from build123d import *

# Parameters (mm, degrees)
IZIM1_W                     = 20
IZIM1_H                     = 20
Y_KSEKLIK_EKSTR_ZYON1_DEPTH = 10
BO_ALTMA1_T                 = -1
IZIM2_R                     = 20
KES_EKSTR_ZYON1_DEPTH       = 29
Y_KSEKLIK_EKSTR_ZYON2_DEPTH = 4
Y_KSEKLIK_EKSTR_ZYON3_REACH = 29.441
IZIM4_W                     = 8
IZIM4_H                     = 1.735346843
Y_KSEKLIK_EKSTR_ZYON4_START = -10.860571
IZIM6_W                     = 1.735346843
IZIM6_H                     = 8
Y_KSEKLIK_EKSTR_ZYON4_DEPTH = 10.860571
BO_ALTMA2_START             = 1.404082058
BO_ALTMA2_OUTLINE_W         = 9.860571099
BO_ALTMA2_OUTLINE_H         = 6
BO_ALTMA2_DEPTH             = 9.595917942
BO_ALTMA2_START_2           = 10
BO_ALTMA2_2_OUTLINE_W       = 1.735346843
BO_ALTMA2_2_OUTLINE_H       = 6
BO_ALTMA2_2_DEPTH           = 1
IZIM7_W                     = 1
IZIM7_H                     = 6
Y_KSEKLIK_EKSTR_ZYON5_DEPTH = 1.735346843
RADYUS1_R                   = 1
RADYUS2_R                   = 1
IZIM8_W                     = 12.756136784
IZIM8_H                     = 3
KES_EKSTR_ZYON2_DEPTH       = 10
RADYUS3_R                   = 0.5


# Read off the part's stored shape, not the designer's step: __ İç Boşaltma2
with BuildPart() as part:
    # Çizim1 → Yükseklik-Ekstrüzyon1 (new, symmetric)
    with BuildSketch(Plane.XY):
        Rectangle(IZIM1_W, IZIM1_H)
    extrude(amount=Y_KSEKLIK_EKSTR_ZYON1_DEPTH, both=True)

    # İç Boşaltma1
    bo_altma1_openings = [part.faces().sort_by_distance(p)[0] for p in [
        (0, -10, 0),
    ]]
    offset(amount=BO_ALTMA1_T, openings=bo_altma1_openings, kind=Kind.INTERSECTION)

    # Çizim2 → Kes-Ekstrüzyon1 (cut)
    with BuildSketch(Plane.XY.offset(10)):
        with Locations((20, -20)):
            Circle(IZIM2_R)
    extrude(amount=-KES_EKSTR_ZYON1_DEPTH, mode=Mode.SUBTRACT)

    # Çizim3 → Yükseklik-Ekstrüzyon2 (add, symmetric)
    with BuildSketch(Plane.XY):
        Polygon((10, -2.139428901), (12, -2.139428901), (12, -13), (2.139428901, -13), (2.139428901, -11), (2.139428901, -2.139428901), align=None)
    extrude(amount=Y_KSEKLIK_EKSTR_ZYON2_DEPTH, both=True)

    # Çizim4 → Yükseklik-Ekstrüzyon3 (add, up to next)
    with BuildSketch(Plane(origin=(12, 0, 0), x_dir=(0, 0, -1), z_dir=(1, 0, 0)), mode=Mode.PRIVATE) as y_kseklik_ekstr_zyon3_sk1:
        with Locations((0, -1.27175548)):
            Rectangle(IZIM4_W, IZIM4_H)
    y_kseklik_ekstr_zyon3_tool1 = extrude(y_kseklik_ekstr_zyon3_sk1.sketch, amount=-Y_KSEKLIK_EKSTR_ZYON3_REACH, mode=Mode.PRIVATE) - part.part
    add(y_kseklik_ekstr_zyon3_tool1.solids().sort_by_distance((12, -1.271755, 0))[0])

    # Çizim6 → Yükseklik-Ekstrüzyon4 (add)
    with BuildSketch(Plane.XZ.offset(13).offset(Y_KSEKLIK_EKSTR_ZYON4_START)):
        with Locations((1.27175548, 0)):
            Rectangle(IZIM6_W, IZIM6_H)
    extrude(amount=Y_KSEKLIK_EKSTR_ZYON4_DEPTH)

    # İç Boşaltma2 outline → İç Boşaltma2 (cut)
    with BuildSketch(Plane.YZ.offset(BO_ALTMA2_START)):
        with Locations((-8.06971445, 0)):
            Rectangle(BO_ALTMA2_OUTLINE_W, BO_ALTMA2_OUTLINE_H)
    extrude(amount=BO_ALTMA2_DEPTH, mode=Mode.SUBTRACT)

    # Bo_altma2 2 outline → Bo_altma2 2 (cut)
    with BuildSketch(Plane.YZ.offset(BO_ALTMA2_START_2)):
        with Locations((-2.27175548, 0)):
            Rectangle(BO_ALTMA2_2_OUTLINE_W, BO_ALTMA2_2_OUTLINE_H)
    extrude(amount=BO_ALTMA2_2_DEPTH, mode=Mode.SUBTRACT)

    # Çizim7 → Yükseklik-Ekstrüzyon5 (add)
    with BuildSketch(Plane.XZ.offset(3.139428901)):
        with Locations((10.5, 0)):
            Rectangle(IZIM7_W, IZIM7_H)
    extrude(amount=-Y_KSEKLIK_EKSTR_ZYON5_DEPTH)

    # Radyus1
    radyus1_edges = [part.edges().sort_by_distance(p)[0] for p in [
        (-10, 0, 10),
        (10, 3.660254038, -10),
        (10, 3.660254038, 10),
        (-10, 0, -10),
        (0, 10, -10),
        (0, 10, 10),
        (-10, 10, 0),
        (10, 10, 0),
    ]]
    fillet(radyus1_edges, radius=RADYUS1_R)

    # Radyus2
    radyus2_edges = [part.edges().sort_by_distance(p)[0] for p in [
        (-3.160254038, -10, 10),
        (-9.707106781, -10, 9.707106781),
        (-3.160254038, -10, -10),
        (-9.707106781, -10, -9.707106781),
        (-10, -10, 0),
    ]]
    fillet(radyus2_edges, radius=RADYUS2_R - 0.0001)  # a hair under: the kernel refuses the full size

    # Çizim8 → Kes-Ekstrüzyon2 (cut)
    with BuildSketch(Plane.XY.offset(4)):
        with Locations((6.78215045, -13.5)):
            Rectangle(IZIM8_W, IZIM8_H)
    extrude(amount=-KES_EKSTR_ZYON2_DEPTH, mode=Mode.SUBTRACT)

    # Radyus3
    radyus3_edges = [part.edges().sort_by_distance(p)[0] for p in [
        (12, -6.202041029, -4),
        (12, -6.202041029, 4),
        (6.202041029, -12, 4),
        (12, -12, 0),
        (6.202041029, -12, -4),
        (0.404082058, -12, 0),
        (12, -0.404082058, 0),
        (0.404082058, -7.0697145, -4),
        (0.404082058, -7.0697145, 4),
    ]]
    fillet(radyus3_edges, radius=RADYUS3_R)


solid = part.part
The model under review builds one solid part; all positions refer to its coordinate system, in mm. A direction names the side the tool comes from. Round coordinates to 2 decimals unless told otherwise and drop trailing zeros. Order: outer loops, then holes, each group sorted by start corner. A loop starts at its lowest first (then second) coordinate and runs counter-clockwise, first axis right, second up. Notation, with made-up numbers: (-6, 10) -> (44, 10) arc R24 cw to (44, 40) -> close; hole circle Ø4 at (-4.5, -5.5). An arc over 180 degrees is marked (long way). Return JSON: item names as keys, results as strings.
1. Take a section at D-D (x = 8.5). Write out the cut boundary in (y, z), then the cut area to 3 significant figures.
Answer block:
{"outline": "(-12, -3.5) arc R0.5 ccw to (-11.5, -4) -> (-2.14, -4) -> (-2.14, 4) -> (-11.5, 4) arc R0.5 ccw to (-12, 3.5) -> (-12, 3) -> (-3.14, 3) -> (-3.14, -3) -> (-12, -3) -> close; (-3.64, -10) -> (9, -10) arc R1 ccw to (10, -9) -> (10, 9) arc R1 ccw to (9, 10) -> (-3.64, 10) -> (-3.64, 9) -> (9, 9) -> (9, -9) -> (-3.64, -9) -> close", "area": "70.5 mm²"}
2. For L1, parallel to Z at x = 4.75, y = -5; L2, parallel to Z at x = 5.5, y = -2.5; L3, parallel to X at y = -3.5, z = 3.5, list the stretches that pass through material, from the lowest coordinate up. Write a range as [from, to].
Answer block:
{"L1": "z = [-10, -9], [-4, -3], [3, 4], [9, 10]", "L2": "z = [-10, -9], [-4, 4], [9, 10]", "L3": "x = [-10, -9], [0.4, 12]"}
3. For faces 1 (the face through (7.31, -4.54, 9.24)), 2 (the face through (11, -0.404, 0)), 3 (the face through (-9, -1, 0)), list the 3-axis set-ups (+Z, -Z, +X, -X, +Y, -Y) from which the entire face can be reached by the end or side of a thin tool; tool diameter is ignored.
Answer block:
{"face 1": "+Z, +X, -Y", "face 2": "+Z, -Z, +X, +Y", "face 3": "-Y"}
4. Insertion check: P1, Ø6, axis at y = 5, z = -5.5, coming from the +X side; P2, Ø5.5, axis at x = -2, z = -2, coming from the -Y side; P3, Ø2, axis at x = -3.5, z = -6, coming from the -Y side. Each pin has a flat end and moves straight along its axis. Give the tip position at first contact, or say it passes through.
Answer block:
{"P1": "stops at x = 10", "P2": "stops at y = -11.98", "P3": "stops at y = 9"}
5. Take a section at C-C (y = 3). Write out the cut boundary in (x, z).
Answer block:
{"outline": "(-10, -9) arc R1 ccw to (-9, -10) -> (9, -10) arc R1 ccw to (10, -9) -> (10, 9) arc R1 ccw to (9, 10) -> (-9, 10) arc R1 ccw to (-10, 9) -> close; hole (-9, -9) -> (9, -9) -> (9, 9) -> (-9, 9) -> close"}
6. The part is to be moulded in two halves that separate along Y. For faces 4 (the face through (0, 0, -9)), 5 (the face through (5, -2.139, 0)), 6 (the face through (0.126, 9.699, -9.715)), say which applies: +Y half, -Y half, draft (parallel to the pull), parting line (faces both ways), or undercut.
Answer block:
{"face 4": "draft", "face 5": "undercut", "face 6": "+Y half"}
